Geometry: see drawing. Coordinates: mm, zero at the bounding-box minimum. A direction names the side the tool comes from. Give positions to 0.01 mm unless a question says otherwise; leave off trailing zeros. Write each loop counter-clockwise with the first axis right and the second up, starting at its lowest first coordinate (ties: lowest second). Pieces come first, ordered by that corner, then holes. Notation, with made-up numbers: M -16.5,13.25 L -8.5,13.25 A29 ccw -8.5,36.25 Z; hole C -32.75,-15.5 d5. An arc over 180 degrees is marked long. Use a Markdown table: item, result. Add a question column.
1) Section C-C on z = 1.5. Return the cut outline in (x, y), then the cut area to 3 significant figures.
2) Line query: line 1 (Y direction, x = 18.85, z = 7.6); line 2 (Z direction, x = 21.5, y = 2); line 3 (X direction, y = 29, z = 1.25). Output: solid intervals per line, ascending.
3) Section D-D on z = 3.5. Return the cut outline in (x, y), then the cut area to 3 significant figures.
4) Set-up query: the marked faces 1 and 2. Return all of +Z, -Z, +X, -X, +Y, -Y with unobstructed straight access to the full face (end or side cutting, diameter ignored); none if empty.
5) Pin query (flat end, axial travel): pin 1 (5 mm diameter, centred on y = 15.5, z = 6.5, fed in from +X); pin 2 (6 mm diameter, centred on x = 9.5, y = 5, fed in from +Z); pin 3 (1 mm diameter, centred on y = 22.5, z = 3, fed in from -X); pin 4 (1.5 mm diameter, centred on x = 33.5, y = 13, fed in from -Z). Return the tip coordinate at first contact, or that it passes through.
6) Section A-A on x = 18.85. Return the cut outline in (y, z).
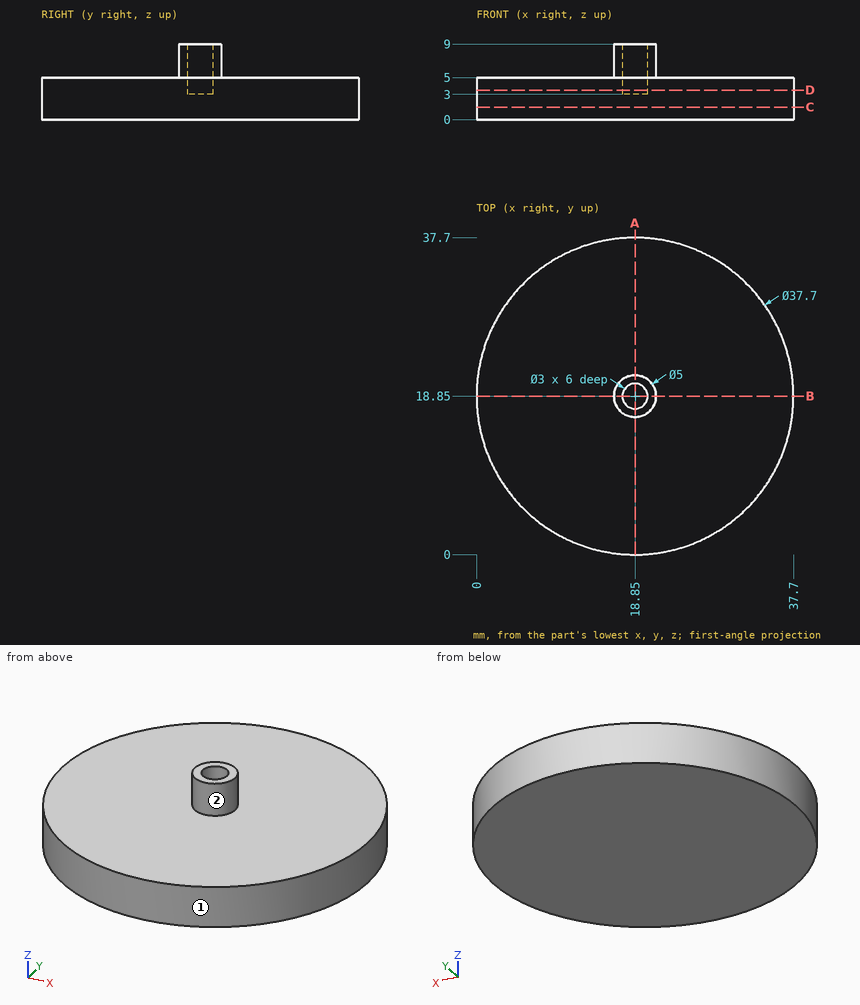
Found:
| question | item | result |
|---|---|---|
| 1 | outline | C 18.85,18.85 d37.7 |
| 1 | area | 1,120 mm² |
| 2 | line 1 | 16.35 to 17.35, 20.35 to 21.35 |
| 2 | line 2 | 0 to 5 |
| 2 | line 3 | 2.97 to 34.73 |
| 3 | outline | C 18.85,18.85 d37.7; hole C 18.85,18.85 d3 |
| 3 | area | 1,110 mm² |
| 4 | face 1 | +Z, -Z |
| 4 | face 2 | +Z |
| 5 | pin 1 | x = 37.65 |
| 5 | pin 2 | z = 5 |
| 5 | pin 3 | x = 0.27 |
| 5 | pin 4 | z = 0 |
| 6 | outline | M 0,0 L 37.7,0 L 37.7,5 L 21.35,5 L 21.35,9 L 20.35,9 L 20.35,3 L 17.35,3 L 17.35,9 L 16.35,9 L 16.35,5 L 0,5 Z |
